The listing builds one solid part. Answer for the finished solid, in the listing's coordinates (mm). A direction names the side the tool comes from. Coordinates: 2 decimals unless noted, no trailing zeros. Write each loop counter-clockwise with the first axis right and the second up, starting at its lowest first coordinate (ties: lowest second). Pieces come first, ordered by that corner, then holes.
(1) Which of the six approach directions +Z, -Z, +X, -X, +Y, -Y give full straight-line access (tool end or side, diameter ignored) to faces 1 (the flat face through (174, -6.35, 165)), 2 (the flat face through (169, -12.7, 90))?
(2) For a pull along Z with two mould halves and no side action, classify faces 3 (the flat face through (342.9, -6, 88)), 4 (the flat face through (169, -6, 177.8)), 5 (the flat face through (6.35, -3, 13)) as +Z half, -Z half, draft (parallel to the pull), parting line (faces both ways), or undercut.
(3) Straight lines are drawn through the part: line 1 (Z direction, x = 223, y = -2); line 2 (X direction, y = -5.75, z = 163); line 3 (Y direction, x = 110, z = 18.5). For each, find the intervals that lie inside material, in ascending order.
(4) The part is cut by section A-A on y = -2. Determine the outline of the cut face in (x, z), plus the area to 3 significant figures.
(5) Given P1, Ø6.5, axis at x = 107.5, z = 166.5, coming from the +Y side, flat-ended and moving along its own axis, determine where the tip first touches the part or whether it passes through.
(6) The part is cut by section B-B on x = 59.5. Determine the outline of the cut face in (y, z), plus the area to 3 significant figures.
from build123d import *

# Parameters (mm, degrees)
F0_W     = 342.9
F0_H     = 177.8
F1_DEPTH = 12.7
F2_W     = 330.2
F2_H     = 12.7
F3_DEPTH = 6.35
F4_W     = 330.2
F4_H     = 12.7
F5_DEPTH = 6.35


with BuildPart() as f1:
    # F0 (on Front) → F1 (new body)
    with BuildSketch(Plane.XZ):
        with Locations((171.45, 88.9)):
            Rectangle(F0_W, F0_H)
    extrude(amount=F1_DEPTH)

    # F2 (on face) → F3 (cut)
    with BuildSketch(Plane(origin=(0, 0, 0), x_dir=(-1, 0, 0), z_dir=(0, 1, 0))):
        with Locations((-171.45, 12.7)):
            Rectangle(F2_W, F2_H)
    extrude(amount=-F3_DEPTH, mode=Mode.SUBTRACT)

    # F4 (on face) → F5 (cut)
    with BuildSketch(Plane(origin=(0, 0, 0), x_dir=(-1, 0, 0), z_dir=(0, 1, 0))):
        with Locations((-171.45, 165.1)):
            Rectangle(F4_W, F4_H)
    extrude(amount=-F5_DEPTH, mode=Mode.SUBTRACT)


solid = f1.part
Model answer:
1. face 1: +Y
1. face 2: +Z, -Z, +X, -X, -Y
2. face 3: draft
2. face 4: +Z half
2. face 5: undercut
3. line 1: z = 0 to 6.35, 19.05 to 158.75, 171.45 to 177.8
3. line 2: x = 0 to 6.35, 336.55 to 342.9
3. line 3: y = -12.7 to -6.35
4. outline: (0, 0) - (342.9, 0) - (342.9, 177.8) - (0, 177.8) - close; hole (6.35, 6.35) - (336.55, 6.35) - (336.55, 19.05) - (6.35, 19.05) - close; hole (6.35, 158.75) - (336.55, 158.75) - (336.55, 171.45) - (6.35, 171.45) - close
4. area: 52,600 mm2
5. P1: stops at y = -6.35
6. outline: (-12.7, 0) - (0, 0) - (0, 6.35) - (-6.35, 6.35) - (-6.35, 19.05) - (0, 19.05) - (0, 158.75) - (-6.35, 158.75) - (-6.35, 171.45) - (0, 171.45) - (0, 177.8) - (-12.7, 177.8) - close
6. area: 2,100 mm2
